from build123d import *

# Parameters (mm, degrees)
F0_R      = 6.35
F1_DEPTH  = 6.35
F2_R      = 15.875
F3_DEPTH  = 44.45
F4_SIZE   = 5.08
F5_SIZE   = 5.08
F6_R      = 10.6348002919
F7_DEPTH  = 6.35
F8_R      = 4.7625
F9_DEPTH  = 31.75
F11_R     = 6.35
F12_DEPTH = 6.35
F13_R     = 6.35
F14_DEPTH = 31.75
F15_R     = 15.875
F16_DEPTH = 6.35
F20_R     = 11.1125
F21_DEPTH = 9.525
F22_R     = 4.7625
F23_DEPTH = 31.75


with BuildPart() as f1:
    # F0 (on Top) → F1 (new body)
    with BuildSketch(Plane.XY):
        with Locations((-69.4737806916, -28.0783642083)):
            Circle(F0_R)
    extrude(amount=F1_DEPTH)

    # F2 (on face) → F3 (join)
    with BuildSketch(Plane.XY.offset(6.35)):
        with Locations((-69.4737806916, -28.0783642083)):
            Circle(F2_R)
    extrude(amount=F3_DEPTH)

    # F4
    f4_edges = [f1.edges().sort_by_distance(p)[0] for p in [
        (-53.598781, -28.078364, 28.575),
        (-85.348781, -28.078364, 6.35),
        (-85.348781, -28.078364, 50.8),
    ]]
    chamfer(f4_edges, length=F4_SIZE)

    # F5
    f5_edges = [f1.edges().sort_by_distance(p)[0] for p in [
        (-53.598781, -28.078364, 28.575),
        (-85.348781, -28.078364, 11.43),
        (-85.348781, -28.078364, 45.72),
    ]]
    chamfer(f5_edges, length=F5_SIZE)

    # F6 (on face) → F7 (cut)
    with BuildSketch(Plane.XY.offset(50.8)):
        with Locations((-69.4737806916, -28.0783642083)):
            Circle(F6_R)
    extrude(amount=-F7_DEPTH, mode=Mode.SUBTRACT)

    # F8 (on face) → F9 (cut)
    with BuildSketch(Plane.XY.offset(44.45)):
        with Locations((-69.4737806916, -28.0783642083)):
            Circle(F8_R)
    extrude(amount=-F9_DEPTH, mode=Mode.SUBTRACT)


with BuildPart() as f12:
    # F11 (on Top) → F12 (new body)
    with BuildSketch(Plane.XY):
        with Locations((-63.7479051948, -45.2827736735)):
            Circle(F11_R)
    extrude(amount=F12_DEPTH)

    # F13 (on face) → F14 (join)
    with BuildSketch(Plane.XY.offset(6.35)):
        with Locations((-63.7479051948, -45.2827736735)):
            Circle(F13_R)
    extrude(amount=F14_DEPTH)

    # F15 (on face) → F16 (join)
    with BuildSketch(Plane.XY.offset(38.1)):
        with Locations((-63.7479051948, -45.2827736735)):
            Circle(F15_R)
    extrude(amount=F16_DEPTH)


with BuildPart() as f18:
    # F17 (on Front) → F18 (revolve)
    with BuildSketch(Plane.XZ):
        Polygon((28.1351623714, 49.0950892346), (23.3591329306, 39.5371243358), (32.8976623714, 10.9950892346), (32.8976623714, 4.6450892346), (39.2476623714, 4.6450892346), (39.2476623714, 49.0950892346), align=None)
    revolve(axis=Axis((39.2476623714, 0, 26.8700892346), (0, 0, 1)))

    # F20 (on face) → F21 (cut)
    with BuildSketch(Plane.XY.offset(49.0950892346)):
        with Locations((39.2476623714, 0)):
            Circle(F20_R)
    extrude(amount=-F21_DEPTH, mode=Mode.SUBTRACT)

    # F22 (on face) → F23 (cut)
    with BuildSketch(Plane.XY.offset(39.5700892346)):
        with Locations((39.2476623714, 0)):
            Circle(F22_R)
    extrude(amount=-F23_DEPTH, mode=Mode.SUBTRACT)


solid = f18.part
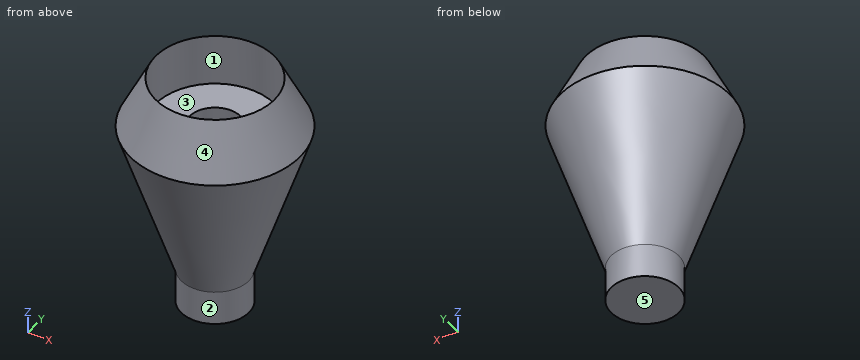
Source: CAD feature listing. Evaluate the final solid. Frame: model axes, mm. Face numbers are marked on the shaded views. A direction names the side the tool comes from. Coordinates: 2 decimals unless noted, no trailing zeros. Order: outer loops, then holes, each group sorted by start corner. A loop starts at its lowest first (then second) coordinate and runs counter-clockwise, first axis right, second up. Notation, with made-up numbers: M -6,35.25 L 24,35.25 A26 cw 24,67.25 Z; hole C 52.5,45 d11. An arc over 180 degrees is marked long. Write each question's results on one line, items separated by ' | '. Start each with the question number.
Item 1: Line query: probe 1 along X at (y, z) = (0, 43.5); probe 2 along X at (y, z) = (0, 43); probe 3 along Y at (x, z) = (36.5, 38). Output: solid intervals per line, ascending.
Item 2: First-contact query: pin 1 Ø10 at (x, z) = (42, 12) entering from -Y; pin 2 Ø8 at (y, z) = (0.5, 20.5) entering from -X; pin 3 Ø4 at (y, z) = (7, 29) entering from -X. Flat tips, straight axial feed; report the tip coordinate or a pass-through.
Item 3: Set-up query: the marked faces 1 and 2. Return all of +Z, -Z, +X, -X, +Y, -Y with unobstructed straight access to the full face (end or side cutting, diameter ignored); none if empty.
Item 4: Cut plane C-C (z = 32). Return loops of the section in (x, y) (1 decimal).
Item 5: Cut plane A-A (y = 0). Return loops of the section in (x, z).
Item 6: Draft query along Y for the marked faces 3, 4 and 5. Return one class per face: pulls with the +Y half, pulls with the -Y half, needs draft (parallel to the pull), parting line crosses it, or undercut.
Checked values:
1) probe 1: x = 25.34 to 28.14, 50.36 to 53.16 | probe 2: x = 25.09 to 28.14, 50.36 to 53.41 | probe 3: y = -15.13 to -3.89, 3.89 to 15.13
2) pin 1: stops at y = -8.19 | pin 2: stops at x = 28.39 | pin 3: stops at x = 27.68
3) face 1: +Z | face 2: -Z
4) outline: C 39.2,0 d26.7; hole C 39.2,0 d9.5
5) outline: M 23.36,39.54 L 32.9,11 L 32.9,4.65 L 45.6,4.65 L 45.6,11 L 55.14,39.54 L 50.36,49.1 L 50.36,39.57 L 44.01,39.57 L 44.01,7.82 L 34.49,7.82 L 34.49,39.57 L 28.14,39.57 L 28.14,49.1 Z
6) face 3: undercut | face 4: parting line crosses it | face 5: needs draft
